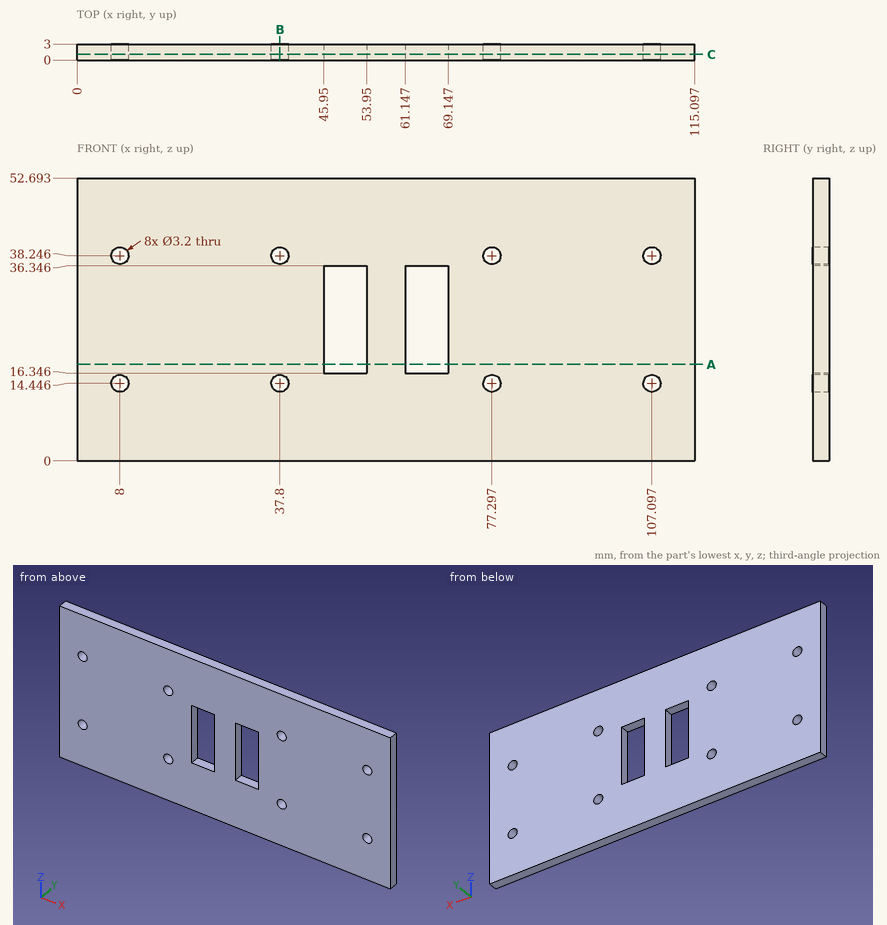
Part print with two shaded views. Sizes in mm from the minimum x, y, z corner. Round coordinates to 2 decimals unless told otherwise and drop trailing zeros. Order: outer loops, then holes, each group sorted by start corner. A loop starts at its lowest first (then second) coordinate and runs counter-clockwise, first axis right, second up. Notation, with made-up numbers: (1.25, 17.5) - (55.25, 17.5) arc R14 cw to (55.25, 25.5) - close; hole circle Ø2 at (-6, 79). An arc over 180 degrees is marked (long way). Return JSON: item names as keys, results as strings.
(1) Cut at A-A (z = 18). Give the cut face in (x, y), then the cut area to 3 significant figures.
Answer key:
{"outline": "(0, 0) - (45.95, 0) - (45.95, 3) - (0, 3) - close; (53.95, 0) - (61.15, 0) - (61.15, 3) - (53.95, 3) - close; (69.15, 0) - (115.1, 0) - (115.1, 3) - (69.15, 3) - close", "area": "297 mm^2"}
(2) Cut at B-B (x = 37.8). Give the cut face in (y, z).
Answer key:
{"outline": "(0, 0) - (3, 0) - (3, 12.85) - (0, 12.85) - close; (0, 16.05) - (3, 16.05) - (3, 36.65) - (0, 36.65) - close; (0, 39.85) - (3, 39.85) - (3, 52.69) - (0, 52.69) - close"}
(3) Cut at C-C (y = 1.05). State how many separate pieces and enclosed holes the cut face has, then the cut area to 3 significant figures.
Answer key:
{"separate pieces": "1", "enclosed holes": "10", "area": "5,680 mm^2"}
(4) Wall check: probe 1 along X at (y, z) = (1.4, 26); probe 2 along Z at (x, y) = (8, 1.2); probe 3 along Z at (x, y) = (63, 1.65). Give the ranges that are in metal, low to high. Write a range as from..to.
Answer key:
{"probe 1": "x = 0..45.95, 53.95..61.15, 69.15..115.1", "probe 2": "z = 0..12.85, 16.05..36.65, 39.85..52.69", "probe 3": "z = 0..16.35, 36.35..52.69"}
